Build history of the part. All positions in model axes, mm. Face numbers are marked on the shaded views. A direction names the side the tool comes from. Give positions to 0.01 mm unless a question says otherwise; leave off trailing zeros. Loops run counter-clockwise (first coordinate to the right, second up) from the corner with the lowest first, then second, coordinate; pieces in that order, holes last. Notation, with made-up numbers: (-11.75, 60.5) -> (-2.75, 60.5) arc R26 ccw to (-2.75, 86.5) -> close; hole circle Ø10 at (1, 23.5). An arc over 180 degrees is marked (long way). Answer as a JSON object with one key per item and string values. Group by question number.
Q1. Band-saw the part on A-A, the plane y = -25. Write the cut outline in (x, z), plus the area to 3 significant figures.
Q2. Wall check: probe 1 along Y at (x, z) = (0, 1.6); probe 2 along Y at (x, z) = (-13, 0.45); probe 3 along X at (y, z) = (14, 1.55). Give the ranges that are in metal, low to high. Write a range as from..to.
Q3. Band-saw the part on C-C, the plane z = 5.4. Count the separate pieces of the cut face and the enclosed holes in it, plus the area to 3 significant figures.
Q4. Two-plate mould, pull along X, no slides. Class the marked faces 5, 6, 7 and 8: pulls with the +X half, pulls with the -X half, needs draft (parallel to the pull), parting line crosses it, or undercut.
Q5. Band-saw the part on B-B, the plane x = 0. Write the cut outline in (y, z), plus the area to 3 significant figures.
Q6. Drop a flat-ended pin along its axis: pin 1 (1.8 mm diameter, centred on y = -22.5, z = 3, fed in from -X). Give the stop position or say it passes through.
Q7. Band-saw the part on D-D, the plane x = -13. Write the cut outline in (y, z).
Q8. Tool access for the marked faces 1, 2, 3 and 4: list every direction of +Z, -Z, +X, -X, +Y, -Y with a clear straight run to the whole face (end or side of a thin tool).
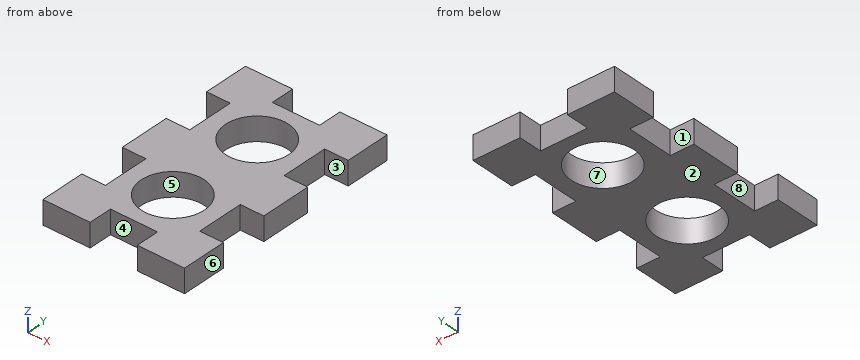
Autodesk Inventor part; units mm, degrees
ref_plane "YZ Plane" through (0, 0, 0) normal (1, 0, 0) x (0, 1, 0)
ref_plane "XZ Plane" through (0, 0, 0) normal (0, 1, 0) x (-1, 0, 0)
ref_plane "XY Plane" through (0, 0, 0) normal (0, 0, 1) x (1, 0, 0)
sketch "Sketch1" plane through (0, 0, 0) normal (0, 0, 1) x (1, 0, 0)
  circle A0 centre (0, 0) radius 8
  circle A1 centre (0, -25) radius 8
  line L0 (0, 0) -> (0, -25) construction
  line L1 (-18, 17.5) -> (18, 17.5)
  line L2 (18, 17.5) -> (18, -42.5)
  line L3 (18, -42.5) -> (-18, -42.5)
  line L4 (-18, -42.5) -> (-18, 17.5)
  line L5 (-18, 17.5) -> (18, -42.5) construction
  line L6 (18, 17.5) -> (-18, -42.5) construction
  line L7 (-6, 17.5) -> (6, 17.5)
  line L8 (6, 17.5) -> (6, 11.5)
  line L9 (6, 11.5) -> (-6, 11.5)
  line L10 (-6, 11.5) -> (-6, 17.5)
  line L11 (-6, -42.5) -> (6, -42.5)
  line L12 (6, -42.5) -> (6, -36.5)
  line L13 (6, -36.5) -> (-6, -36.5)
  line L14 (-6, -36.5) -> (-6, -42.5)
  line L15 (-18, -31) -> (-12, -31)
  line L16 (-12, -31) -> (-12, -19)
  line L17 (-12, -19) -> (-18, -19)
  line L18 (-18, -19) -> (-18, -31)
  line L19 (-18, -6) -> (-12, -6)
  line L20 (-12, -6) -> (-12, 6)
  line L21 (-12, 6) -> (-18, 6)
  line L22 (-18, 6) -> (-18, -6)
  line L23 (18, -6) -> (12, -6)
  line L24 (12, -6) -> (12, 6)
  line L25 (12, 6) -> (18, 6)
  line L26 (18, 6) -> (18, -6)
  line L27 (18, -31) -> (12, -31)
  line L28 (12, -31) -> (12, -19)
  line L29 (12, -19) -> (18, -19)
  line L30 (18, -19) -> (18, -31)
  point P0 (0, -12.5)
  point P1 (0, 11.5)
  point P2 (0, 17.5)
  point P3 (12, 0)
  point P4 (-12, 0)
  point P5 (-12, -25)
  point P6 (12, -25)
  dimension "d0" = 16
  dimension "d1" = 25
  dimension "d2" = 36
  dimension "d3" = 60
  dimension "d4" = 12
  dimension "d5" = 6
extrude "Plate1" add sketch "Sketch1" along normal blind 6 contours L1 L10 L9 L8 L2 L25 L24 L23 L29 L28 L27 L3 L12 L13 L14 L4 L15 L16 L17 L19 L20 L21
equation "\"d7\" = Thickness"
equation "\"BendRadius\" = Thickness"
equation "\"BendReliefWidth\" = Thickness"
equation "\"BendReliefDepth\" = 0.5 * Thickness"
equation "\"CornerReliefSize\" = 4 * Thickness"
equation "\"MinimumRemnant\" = 2 * Thickness"
equation "\"TransitionRadius\" = BendRadius"
equation "\"JacobiRadiusSize\" = BendRadius"
equation "\"GapSize\" = Thickness"
properties part number "voorkant knoppendoosje" material "Wood (Birch)"
Worked answers:
{
 "1": {"outline": "(-12, 0) -> (-8, 0) -> (-8, 6) -> (-12, 6) -> close; (8, 0) -> (12, 0) -> (12, 6) -> (8, 6) -> close", "area": "48.0 mm2"},
 "2": {"probe 1": "-36.5..-33, -17..-8, 8..11.5", "probe 2": "-42.5..-31, -19..-6, 6..17.5", "probe 3": "-18..-6, 6..18"},
 "3": {"separate pieces": "1", "enclosed holes": "2", "area": "1,330 mm2"},
 "4": {"face 5": "undercut", "face 6": "pulls with the +X half", "face 7": "undercut", "face 8": "pulls with the -X half"},
 "5": {"outline": "(-36.5, 0) -> (-33, 0) -> (-33, 6) -> (-36.5, 6) -> close; (-17, 0) -> (-8, 0) -> (-8, 6) -> (-17, 6) -> close; (8, 0) -> (11.5, 0) -> (11.5, 6) -> (8, 6) -> close", "area": "96.0 mm2"},
 "6": {"pin 1": "x = -12"},
 "7": {"outline": "(-42.5, 0) -> (-31, 0) -> (-31, 6) -> (-42.5, 6) -> close; (-19, 0) -> (-6, 0) -> (-6, 6) -> (-19, 6) -> close; (6, 0) -> (17.5, 0) -> (17.5, 6) -> (6, 6) -> close"},
 "8": {"face 1": "+Z, -Z, -X", "face 2": "-Z, +X, -X, +Y, -Y", "face 3": "+Z, -Z, +X", "face 4": "+Z, -Z, -Y"}
}
